```python
from build123d import *

# Parameters (mm, degrees)
SKETCH1_R                = 1.35
BOSS_EXTRUDE1_DEPTH      = 3
BOSS_EXTRUDE3_DEPTH      = 3
SKETCH2_R                = 3
SKETCH2_R_2              = 1.35
BOSS_EXTRUDE2_DEPTH      = 3
SKETCH4_R                = 5
SKETCH4_R_2              = 1.65
BOSS_EXTRUDE4_DEPTH      = 6
FILLET1_R                = 10
SKETCH6_R                = 5
SKETCH6_R_2              = 1.65
BOSS_EXTRUDE5_DEPTH      = 6
FILLET2_R                = 10
CIRPATTERN4_COUNT        = 2
FILLET1_OF_CIRPATTERN4_R = 10
FILLET2_OF_MIRROR1_R     = 10


with BuildPart() as part:
    # Sketch1 → Boss-Extrude1 (new body)
    with BuildSketch(Plane(origin=(0, 0, 0), x_dir=(1, 0, 0), z_dir=(0, 1, 0))):
        with BuildLine():
            Line((-39.5, -28), (39.5, -28))
            ThreePointArc((39.5, -28), (41.621320344, -27.121320344), (42.5, -25))
            Line((42.5, -25), (42.5, 25))
            ThreePointArc((42.5, 25), (41.621320344, 27.121320344), (39.5, 28))
            Line((39.5, 28), (-39.5, 28))
            ThreePointArc((-39.5, 28), (-41.621320344, 27.121320344), (-42.5, 25))
            Line((-42.5, 25), (-42.5, -25))
            ThreePointArc((-42.5, -25), (-41.621320344, -27.121320344), (-39.5, -28))
        make_face()
        with Locations(Location((-39, -24.5, 0), (0, 0, 270))):
            Circle(SKETCH1_R, mode=Mode.SUBTRACT)
        with Locations(Location((-39, 24.5, 0), (0, 0, 270))):
            Circle(SKETCH1_R, mode=Mode.SUBTRACT)
        with Locations(Location((19, 24.5, 0), (0, 0, 270))):
            Circle(SKETCH1_R, mode=Mode.SUBTRACT)
        with Locations(Location((19, -24.5, 0), (0, 0, 270))):
            Circle(SKETCH1_R, mode=Mode.SUBTRACT)
    extrude(amount=BOSS_EXTRUDE1_DEPTH)

    # Sketch3 → Boss-Extrude3 (add)
    with BuildSketch(Plane(origin=(0, 3, 0), x_dir=(1, 0, 0), z_dir=(0, 1, 0))):
        Polygon((-3, 3), (-72.5, 3), (-72.5, -3), (-3, -3), (-3, -72.5), (3, -72.5), (3, -3), (72.5, -3), (72.5, 3), (3, 3), (3, 72.5), (-3, 72.5), align=None)
    boss_extrude3 = extrude(amount=-BOSS_EXTRUDE3_DEPTH)

    # Sketch2 → Boss-Extrude2 (add)
    # profile 1 of 4: a face of its own
    with BuildSketch(Plane(origin=(0, 3, 0), x_dir=(1, 0, 0), z_dir=(0, 1, 0))):
        with Locations(Location((-39, -24.5, 0), (0, 0, 90))):
            Circle(SKETCH2_R)
        with Locations(Location((-39, -24.5, 0), (0, 0, 270))):
            Circle(SKETCH2_R_2, mode=Mode.SUBTRACT)
    # profile 2 of 4: a face of its own
    with BuildSketch(Plane(origin=(0, 3, 0), x_dir=(1, 0, 0), z_dir=(0, 1, 0))):
        with Locations(Location((-39, 24.5, 0), (0, 0, 90))):
            Circle(SKETCH2_R)
        with Locations(Location((-39, 24.5, 0), (0, 0, 270))):
            Circle(SKETCH2_R_2, mode=Mode.SUBTRACT)
    # profile 3 of 4: a face of its own
    with BuildSketch(Plane(origin=(0, 3, 0), x_dir=(1, 0, 0), z_dir=(0, 1, 0))):
        with Locations(Location((19, 24.5, 0), (0, 0, 90))):
            Circle(SKETCH2_R)
        with Locations(Location((19, 24.5, 0), (0, 0, 270))):
            Circle(SKETCH2_R_2, mode=Mode.SUBTRACT)
    # profile 4 of 4: a face of its own
    with BuildSketch(Plane(origin=(0, 3, 0), x_dir=(1, 0, 0), z_dir=(0, 1, 0))):
        with Locations(Location((19, -24.5, 0), (0, 0, 90))):
            Circle(SKETCH2_R)
        with Locations(Location((19, -24.5, 0), (0, 0, 270))):
            Circle(SKETCH2_R_2, mode=Mode.SUBTRACT)
    extrude(amount=BOSS_EXTRUDE2_DEPTH)

    # Sketch4 → Boss-Extrude4 (add)
    with BuildSketch(Plane.XY.offset(3)):
        with Locations((-72.5, 5)):
            Circle(SKETCH4_R)
        with Locations((-72.5, 5)):
            Circle(SKETCH4_R_2, mode=Mode.SUBTRACT)
    boss_extrude4 = extrude(amount=-BOSS_EXTRUDE4_DEPTH)

    # Fillet1
    fillet1_edges = [part.edges().sort_by_distance(p)[0] for p in [
        (-67.917424305, 3, 0),
    ]]
    fillet(fillet1_edges, radius=FILLET1_R)

    # Sketch6 → Boss-Extrude5 (add)
    with BuildSketch(Plane(origin=(3, 0, 0), x_dir=(0, 0, -1), z_dir=(1, 0, 0))):
        with Locations((-72.592807544, 4.999138602)):
            Circle(SKETCH6_R)
        with Locations((-72.592807544, 4.999138602)):
            Circle(SKETCH6_R_2, mode=Mode.SUBTRACT)
    boss_extrude5 = extrude(amount=-BOSS_EXTRUDE5_DEPTH)

    # Fillet2
    fillet2_edges = [part.edges().sort_by_distance(p)[0] for p in [
        (0, 3, 68.009856001),
    ]]
    fillet(fillet2_edges, radius=FILLET2_R)

    # CirPattern4: Boss-Extrude3, Boss-Extrude4 ×2 about axis
    cirpattern4_axis = Axis((0, 0, 0), (0, 1, 0))
    add([boss_extrude3.rotate(cirpattern4_axis, i * 360 / CIRPATTERN4_COUNT) for i in range(1, CIRPATTERN4_COUNT)])
    add([boss_extrude4.rotate(cirpattern4_axis, i * 360 / CIRPATTERN4_COUNT) for i in range(1, CIRPATTERN4_COUNT)])

    # Fillet1 of CirPattern4
    fillet1_of_cirpattern4_edges = [part.edges().sort_by_distance(p)[0] for p in [
        (67.917424305, 3, 0),
    ]]
    fillet(fillet1_of_cirpattern4_edges, radius=FILLET1_OF_CIRPATTERN4_R)

    # Mirror1: Boss-Extrude5 across plane
    add(boss_extrude5.mirror(Plane.XY))

    # Fillet2 of Mirror1
    fillet2_of_mirror1_edges = [part.edges().sort_by_distance(p)[0] for p in [
        (0, 3, -68.009856001),
    ]]
    fillet(fillet2_of_mirror1_edges, radius=FILLET2_OF_MIRROR1_R)


solid = part.part
```
Part model, mm, in its own coordinate system. A direction names the side the tool comes from. Round coordinates to 2 decimals unless told otherwise and drop trailing zeros. Write each loop counter-clockwise with the first axis right and the second up, starting at its lowest first coordinate (ties: lowest second). Pieces come first, ordered by that corner, then holes.
Item 1: Probe L1, parallel to X at y = 4.5, z = -24.5; L2, parallel to Z at x = -2.5, y = 9.25; L3, parallel to Z at x = 39.5, y = 1.75. List the from-to ranges inside material, lowest first.
Results:
L1: x = -42 to -40.35, -37.65 to -36, 16 to 17.65, 20.35 to 22
L2: z = -75.23 to -69.96, 69.96 to 75.23
L3: z = -28 to 28
Item 2: Cut at A-A, the plane z = -52.5. Give the cut face in (x, y).
Results:
outline: (-3, 0) - (3, 0) - (3, 3) - (-3, 3) - close
Item 3: Cut at B-B, the plane z = 63.5. Give the cut face in (x, y), plus the area to 3 significant figures.
Results:
outline: (-3, 0) - (3, 0) - (3, 3.67) - (-3, 3.67) - close
area: 22.0 mm2
Item 4: Drop flat-ended pins along their axis: pin 1 Ø1.8 at (x, z) = (19, -25) entering from +Y; pin 2 Ø4 at (y, z) = (6.5, 37.5) entering from -X; pin 3 Ø5 at (y, z) = (4, -45.5) entering from -X; pin 4 Ø4 at (x, z) = (-26, -14.5) entering from +Y. Give the stop position or say it passes through.
Results:
pin 1: stops at y = 6
pin 2: passes through
pin 3: stops at x = -3
pin 4: stops at y = 3
Item 5: Which spindle directions (+Z, -Z, +X, -X, +Y, -Y) get a long thin tool onto all of the face, cutting with end or side? Do faces 1 (the cylindrical face through (0.04, 4.28, 64.8)), 2 (the flat face through (64, 3, -3)), 3 (the flat face through (64, 3, 3)), 4 (the cylindrical face through (-41.974, 4.479, -24.109)). Say none if no direction does.
Results:
face 1: +X, -X, +Y
face 2: -Z, +X, +Y, -Y
face 3: +Z, +X, +Y, -Y
face 4: +Y
Item 6: Two-plate mould, pull along Z, no slides. Class faces 5 (the cylindrical face through (0.042, 4.367, -71.069)), 6 (the cylindrical face through (-41.974, 4.479, 24.891)), 7 (the flat face through (-64, 3, -3)), 8 (the flat face through (3, 2.8, -58.7)): +Z half, -Z half, draft (parallel to the pull), parting line (faces both ways), or undercut.
Results:
face 5: undercut
face 6: undercut
face 7: -Z half
face 8: draft
